```python
from build123d import *

# Parameters (mm, degrees)
SKETCH1_W           = 89
SKETCH1_H           = 134
BOSS_EXTRUDE1_DEPTH = 2.5
SKETCH3_W           = 73.15
SKETCH3_H           = 118.15
SKETCH3_W_2         = 63.15
SKETCH3_H_2         = 108.15
BOSS_EXTRUDE2_DEPTH = 3
CUT_EXTRUDE1_REACH  = 82.829
SKETCH5_W           = 43.701404931
SKETCH5_H           = 35.210158561
FILLET1_R           = 1
SKETCH8_R           = 2.9
CUT_EXTRUDE2_DEPTH  = 2.5
CUT_EXTRUDE3_REACH  = 82.619
SKETCH9_R           = 1.6


with BuildPart() as part:
    # Sketch1 → Boss-Extrude1 (new, symmetric)
    with BuildSketch(Plane(origin=(0, 0, 0), x_dir=(1, 0, 0), z_dir=(0, 1, 0))):
        Rectangle(SKETCH1_W, SKETCH1_H)
    extrude(amount=BOSS_EXTRUDE1_DEPTH, both=True)

    # Sketch3 → Boss-Extrude2 (add)
    with BuildSketch(Plane(origin=(0, 2.5, 0), x_dir=(1, 0, 0), z_dir=(0, 1, 0))):
        Rectangle(SKETCH3_W, SKETCH3_H)
        Rectangle(SKETCH3_W_2, SKETCH3_H_2, mode=Mode.SUBTRACT)
    extrude(amount=BOSS_EXTRUDE2_DEPTH)

    # Sketch5 → Cut-Extrude1 (cut, up to next)
    with BuildSketch(Plane.XZ.offset(2.5), mode=Mode.PRIVATE) as cut_extrude1_sk1:
        with Locations((-9.260550175, 36.46992072)):
            Rectangle(SKETCH5_W, SKETCH5_H)
    cut_extrude1_tool1 = extrude(cut_extrude1_sk1.sketch, amount=-CUT_EXTRUDE1_REACH, mode=Mode.PRIVATE) & part.part
    add(cut_extrude1_tool1.solids().sort_by_distance((-9.26055, -2.5, 36.469921))[0], mode=Mode.SUBTRACT)

    # Fillet1
    fillet1_edges = [part.edges().sort_by_distance(p)[0] for p in [
        (-44.5, 2.5, 0),
        (0, 2.5, 67),
        (-31.11125264, -2.5, 36.46992072),
        (-9.260550175, -2.5, 18.864841439),
        (12.590152291, -2.5, 36.46992072),
        (-9.260550175, -2.5, 54.075),
        (44.5, 2.5, 0),
        (0, -2.5, 67),
        (-44.5, -2.5, 0),
        (0, -2.5, -67),
        (44.5, -2.5, 0),
        (44.5, 0, 67),
        (-44.5, 0, 67),
        (-44.5, 0, -67),
        (44.5, 0, -67),
        (0, 2.5, -67),
    ]]
    fillet(fillet1_edges, radius=FILLET1_R)

    # Sketch8 → Cut-Extrude2 (cut)
    with BuildSketch(Plane.XZ.offset(2.5)):
        with Locations(Location((40.49479618, -62.99479618, 0), (0, 0, 270))):
            Circle(SKETCH8_R)
        with Locations(Location((-40.49479618, -62.99479618, 0), (0, 0, 90))):
            Circle(SKETCH8_R)
        with Locations(Location((40.49479618, 62.99479618, 0), (0, 0, 90))):
            Circle(SKETCH8_R)
        with Locations(Location((-40.49479618, 62.99479618, 0), (0, 0, 270))):
            Circle(SKETCH8_R)
    extrude(amount=-CUT_EXTRUDE2_DEPTH, mode=Mode.SUBTRACT)

    # Sketch9 → Cut-Extrude3 (cut, up to next)
    with BuildSketch(Plane.XZ, mode=Mode.PRIVATE) as cut_extrude3_sk1:
        with Locations(Location((40.49479618, -62.99479618, 0), (0, 0, 270))):
            Circle(SKETCH9_R)
    cut_extrude3_tool1 = extrude(cut_extrude3_sk1.sketch, amount=-CUT_EXTRUDE3_REACH, mode=Mode.PRIVATE) & part.part
    # Sketch9 → Cut-Extrude3 (cut, up to next)
    with BuildSketch(Plane.XZ, mode=Mode.PRIVATE) as cut_extrude3_sk2:
        with Locations(Location((-40.49479618, -62.99479618, 0), (0, 0, 270))):
            Circle(SKETCH9_R)
    cut_extrude3_tool2 = extrude(cut_extrude3_sk2.sketch, amount=-CUT_EXTRUDE3_REACH, mode=Mode.PRIVATE) & part.part
    # Sketch9 → Cut-Extrude3 (cut, up to next)
    with BuildSketch(Plane.XZ, mode=Mode.PRIVATE) as cut_extrude3_sk3:
        with Locations(Location((40.49479618, 62.99479618, 0), (0, 0, 270))):
            Circle(SKETCH9_R)
    cut_extrude3_tool3 = extrude(cut_extrude3_sk3.sketch, amount=-CUT_EXTRUDE3_REACH, mode=Mode.PRIVATE) & part.part
    # Sketch9 → Cut-Extrude3 (cut, up to next)
    with BuildSketch(Plane.XZ, mode=Mode.PRIVATE) as cut_extrude3_sk4:
        with Locations(Location((-40.49479618, 62.99479618, 0), (0, 0, 270))):
            Circle(SKETCH9_R)
    cut_extrude3_tool4 = extrude(cut_extrude3_sk4.sketch, amount=-CUT_EXTRUDE3_REACH, mode=Mode.PRIVATE) & part.part
    add(cut_extrude3_tool1.solids().sort_by_distance((40.494796, 0, -62.994796))[0], mode=Mode.SUBTRACT)
    add(cut_extrude3_tool2.solids().sort_by_distance((-40.494796, 0, -62.994796))[0], mode=Mode.SUBTRACT)
    add(cut_extrude3_tool3.solids().sort_by_distance((40.494796, 0, 62.994796))[0], mode=Mode.SUBTRACT)
    add(cut_extrude3_tool4.solids().sort_by_distance((-40.494796, 0, 62.994796))[0], mode=Mode.SUBTRACT)


solid = part.part
```
CAD build for the part. Positions are in the model's coordinates, mm. A direction names the side the tool comes from. Round coordinates to 2 decimals unless told otherwise and drop trailing zeros. Loops run counter-clockwise (first coordinate to the right, second up) from the corner with the lowest first, then second, coordinate; pieces in that order, holes last. Notation, with made-up numbers: (-22, 14) - (-4, 14) arc R32 cw to (-4, 49) - close; hole circle Ø9 at (75.5, -39). An arc over 180 degrees is marked (long way). Return JSON: item names as keys, results as strings. Group by question number.
Q1. Tool access for faces 4 (the face through (-42, 0, 62)), 5 (the face through (36.575, 4, 1)), 6 (the face through (-1, 4, 59.075)), 7 (the face through (-7, 2, 54.075)), 8 (the face through (12.59, 0, 36)): list every direction of +Z, -Z, +X, -X, +Y, -Y with a clear straight run to the whole face (end or side of a thin tool).
Q2. Two-plate mould, pull along Z, no slides. Class faces 1 (the face through (-1, 4, -59.075)), 2 (the face through (-33, 5.5, -5)), 3 (the face through (31.575, 4, 1)): +Z half, -Z half, draft (parallel to the pull), parting line (faces both ways), or undercut.
Q3. Drill centre lines: line 1 along Z through (x, y) = (-9.5, 3.75) (3 decimals); line 2 along Z through (x, y) = (2, -1.5) (3 decimals); line 3 along X through (y, z) = (4, -30.5) (3 decimals). Where is each one in solid material? Low to high. Write a range as [from, to].
Q4. Flat gauge pins, fed straight in: pin 1 Ø4.5 at (x, z) = (-40.49, -62.99) entering from +Y; pin 2 Ø1 at (y, z) = (2.5, 23.5) entering from +X; pin 3 Ø4 at (x, y) = (18.5, 4) entering from -Z. Where does each tip first touch, or does it go through?
Q5. Band-saw the part on C-C on x = -29. Give the cut face in (y, z) (3 decimals), plus the area to 3 significant figures.
Q6. Band-saw the part on D-D on z = -17. Give the cut face in (x, y) (3 decimals).
Q7. Band-saw the part on B-B on y = 4. Give the cut face in (x, z) (3 decimals), plus the area to 3 significant figures.
Q8. Band-saw the part on A-A on z = 45.5. Give the cut face in (x, y) (3 decimals).
Solutions:
{
 "1": {"face 4": "-Y", "face 5": "+Z, -Z, +X, +Y", "face 6": "+Z, +X, -X, +Y", "face 7": "+Y", "face 8": "+Y, -Y"},
 "2": {"face 1": "-Z half", "face 2": "draft", "face 3": "undercut"},
 "3": {"line 1": "z = [-59.075, -54.075], [54.075, 59.075]", "line 2": "z = [-67, 18.865], [54.075, 67]", "line 3": "x = [-36.575, -31.575], [31.575, 36.575]"},
 "4": {"pin 1": "stops at y = 2.5", "pin 2": "stops at x = 44.37", "pin 3": "stops at z = -66.87"},
 "5": {"outline": "(-2.5, -66) arc R1 ccw to (-1.5, -67) - (1.5, -67) arc R1 ccw to (2.5, -66) - (2.5, -59.075) - (5.5, -59.075) - (5.5, -54.075) - (2.5, -54.075) - (2.5, 18.865) - (-1.5, 18.865) arc R1 ccw to (-2.5, 17.865) - close; (-2.5, 55.075) arc R1 ccw to (-1.5, 54.075) - (5.5, 54.075) - (5.5, 59.075) - (2.5, 59.075) - (2.5, 66) arc R1 ccw to (1.5, 67) - (-1.5, 67) arc R1 ccw to (-2.5, 66) - close", "area": "523 mm^2"},
 "6": {"outline": "(-44.5, -1.5) arc R1 ccw to (-43.5, -2.5) - (43.5, -2.5) arc R1 ccw to (44.5, -1.5) - (44.5, 1.5) arc R1 ccw to (43.5, 2.5) - (36.575, 2.5) - (36.575, 5.5) - (31.575, 5.5) - (31.575, 2.5) - (-31.575, 2.5) - (-31.575, 5.5) - (-36.575, 5.5) - (-36.575, 2.5) - (-43.5, 2.5) arc R1 ccw to (-44.5, 1.5) - close"},
 "7": {"outline": "(-36.575, -59.075) - (36.575, -59.075) - (36.575, 59.075) - (-36.575, 59.075) - close; hole (-31.575, -54.075) - (31.575, -54.075) - (31.575, 54.075) - (-31.575, 54.075) - close", "area": "1,810 mm^2"},
 "8": {"outline": "(-44.5, -1.5) arc R1 ccw to (-43.5, -2.5) - (-32.111, -2.5) arc R1 ccw to (-31.111, -1.5) - (-31.111, 2.5) - (-31.575, 2.5) - (-31.575, 5.5) - (-36.575, 5.5) - (-36.575, 2.5) - (-43.5, 2.5) arc R1 ccw to (-44.5, 1.5) - close; (12.59, -1.5) arc R1 ccw to (13.59, -2.5) - (43.5, -2.5) arc R1 ccw to (44.5, -1.5) - (44.5, 1.5) arc R1 ccw to (43.5, 2.5) - (36.575, 2.5) - (36.575, 5.5) - (31.575, 5.5) - (31.575, 2.5) - (12.59, 2.5) - close"}
}
